from build123d import *

# Parameters (mm, degrees)
SKETCH1_W                     = 304.8
SKETCH1_H                     = 177.8
BOSS_EXTRUDE1_DEPTH           = 14.224
TAP_DRILL_FOR_8_32_TAP1_D     = 3.4544
TAP_DRILL_FOR_8_32_TAP1_DEPTH = 7.874
TAP_DRILL_FOR_8_32_TAP1_TIP   = 1.037806461
TAP_DRILL_FOR_5_40_TAP1_D     = 2.5781
TAP_DRILL_FOR_5_40_TAP1_DEPTH = 7.874
TAP_DRILL_FOR_5_40_TAP1_TIP   = 0.774539381
F_1_4_CLEARANCE_HOLE1_D       = 6.5278


with BuildPart() as part:
    # Sketch1 → Boss-Extrude1 (new body)
    with BuildSketch(Plane.XY):
        Rectangle(SKETCH1_W, SKETCH1_H)
    extrude(amount=BOSS_EXTRUDE1_DEPTH)

    # Tap Drill for #8-32 Tap1
    with Locations(Plane.XY.offset(14.224)):
        with Locations((-41.39, 41.985), (-41.39, -41.985), (-125.36, -41.985), (-125.36, 41.985), (-83.375, 59.2455), (-83.375, -59.2455)):
            Hole(TAP_DRILL_FOR_8_32_TAP1_D / 2, depth=TAP_DRILL_FOR_8_32_TAP1_DEPTH)
            with Locations((0, 0, -(TAP_DRILL_FOR_8_32_TAP1_DEPTH + TAP_DRILL_FOR_8_32_TAP1_TIP / 2))):  # 118° drill point
                Cone(0, TAP_DRILL_FOR_8_32_TAP1_D / 2, TAP_DRILL_FOR_8_32_TAP1_TIP, mode=Mode.SUBTRACT)

    # Tap Drill for #5-40 Tap1
    with Locations(Plane.XY.offset(14.224)):
        with Locations((-83.375, 21.5), (-83.375, -21.5), (54.950719391, 47.625), (99.400719391, 47.625), (99.400719391, -47.625), (54.950719391, -47.625)):
            Hole(TAP_DRILL_FOR_5_40_TAP1_D / 2, depth=TAP_DRILL_FOR_5_40_TAP1_DEPTH)
            with Locations((0, 0, -(TAP_DRILL_FOR_5_40_TAP1_DEPTH + TAP_DRILL_FOR_5_40_TAP1_TIP / 2))):  # 118° drill point
                Cone(0, TAP_DRILL_FOR_5_40_TAP1_D / 2, TAP_DRILL_FOR_5_40_TAP1_TIP, mode=Mode.SUBTRACT)

    # 1/4 Clearance Hole1 (through all)
    with Locations(Plane(origin=(0, 0, 0), x_dir=(1, 0, 0), z_dir=(0, 0, -1))):
        with Locations((-12.7, 0), (12.7, 0)):
            Hole(F_1_4_CLEARANCE_HOLE1_D / 2)


solid = part.part
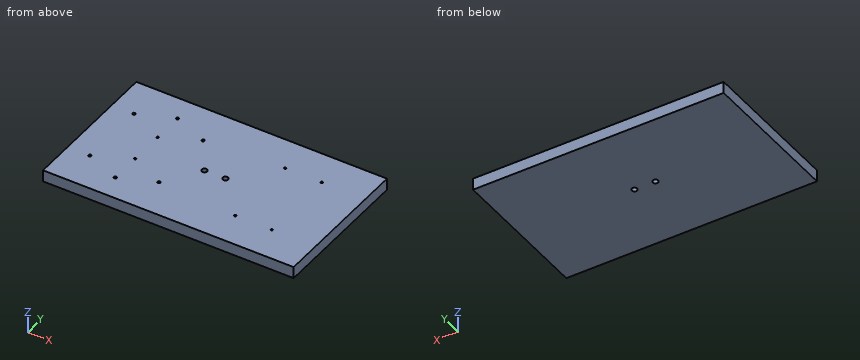
Verification items for the finished model (mm, model axes). Coordinates: 2 decimals unless noted, no trailing zeros. Order: outer loops, then holes, each group sorted by start corner. A loop starts at its lowest first (then second) coordinate and runs counter-clockwise, first axis right, second up.
1. Sectioned sample at B-B, the plane x = -12.7. Record the cut outline in (y, z).
Results found:
outline: (-88.9, 0) - (-3.26, 0) - (-3.26, 14.22) - (-88.9, 14.22) - close; (3.26, 0) - (88.9, 0) - (88.9, 14.22) - (3.26, 14.22) - close
2. Sectioned sample at A-A, the plane y = 0. Record the cut outline in (x, z), and give its area (3 significant figures).
Results found:
outline: (-152.4, 0) - (-15.96, 0) - (-15.96, 14.22) - (-152.4, 14.22) - close; (-9.44, 0) - (9.44, 0) - (9.44, 14.22) - (-9.44, 14.22) - close; (15.96, 0) - (152.4, 0) - (152.4, 14.22) - (15.96, 14.22) - close
area: 4,150 mm2
3. Go/stop test with flat-tipped pins: pin 1 Ø2 at (x, y) = (54.95, -47.62) entering from +Z; pin 2 Ø6 at (x, y) = (12.7, 0) entering from +Z. Record where each tip stops, or that it passes through.
Results found:
pin 1: stops at z = 6.18
pin 2: passes through
4. Scan lines: line 1 (X direction, y = -0.5, z = 13); line 2 (Y direction, x = -125, z = 9.5); line 3 (X direction, y = -21.5, z = 8.5). Record each from-to range of solid material in increasing order.
Results found:
line 1: x = -152.4 to -15.93, -9.47 to 9.47, 15.93 to 152.4
line 2: y = -88.9 to -43.67, -40.3 to 40.3, 43.67 to 88.9
line 3: x = -152.4 to -84.66, -82.09 to 152.4
